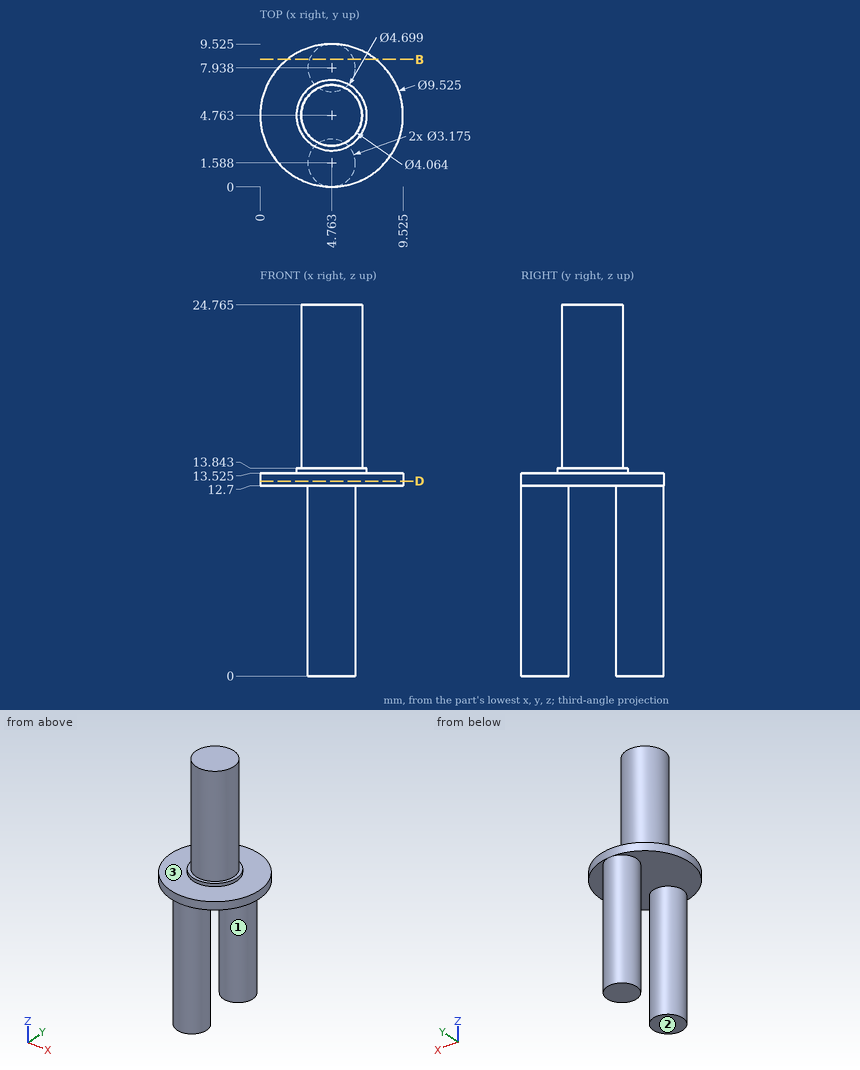
Geometry: see drawing. Coordinates: mm, zero at the bounding-box minimum. A direction names the side the tool comes from. Round coordinates to 2 decimals unless told otherwise and drop trailing zeros. Write each loop counter-clockwise with the first axis right and the second up, starting at its lowest first coordinate (ties: lowest second). Pieces come first, ordered by that corner, then holes. Notation, with made-up numbers: (14.5, -3.5) -> (60.5, -3.5) arc R6 cw to (60.5, 6.5) -> close; hole circle Ø4 at (48, 56). An arc over 180 degrees is marked (long way). Answer as CSV lines item,"result".
1. Section B-B (y = 8.5). Return the cut outline in (x, z) (1 decimal).
Geometry says:
outline,"(1.8, 12.7) -> (3.3, 12.7) -> (3.3, 0) -> (6.2, 0) -> (6.2, 12.7) -> (7.7, 12.7) -> (7.7, 13.5) -> (1.8, 13.5) -> close"
2. Contact query for flat-ended pins moving along their axis: P1, Ø5, axis at x = 8, z = 17, coming from the +Y side (1 decimal); P2, Ø1, axis at x = 8, y = 1.5, coming from the -Z side. Output: stop coordinate, or through.
Geometry says:
P1,"stops at y = 6.7"
P2,"stops at z = 12.7"
3. Reachability of the marked faces 1, 2 and 3 from +Z, -Z, +X, -X, +Y, -Y: full face, straight path, thin tool, end or side. Return the list, or none.
Geometry says:
face 1,"-Z"
face 2,"-Z, +X, -X, +Y, -Y"
face 3,"+Z"
4. Section D-D (z = 13). Return the cut outline in (x, y) (1 decimal).
Geometry says:
outline,"circle Ø9.5 at (4.8, 4.8)"
5. Ray query, L1, parallel to Z at x = 4, y = 4.25 (1 decimal); L2, parallel to Z at x = 4, y = 0.5 (1 decimal); L3, parallel to Y at x = 3.75, z = 13 (1 decimal). Return the intervals inside material, ascending. Write a range as [from, to].
Geometry says:
L1,"z = [12.7, 24.8]"
L2,"z = [0, 13.5]"
L3,"y = [0.1, 9.4]"
